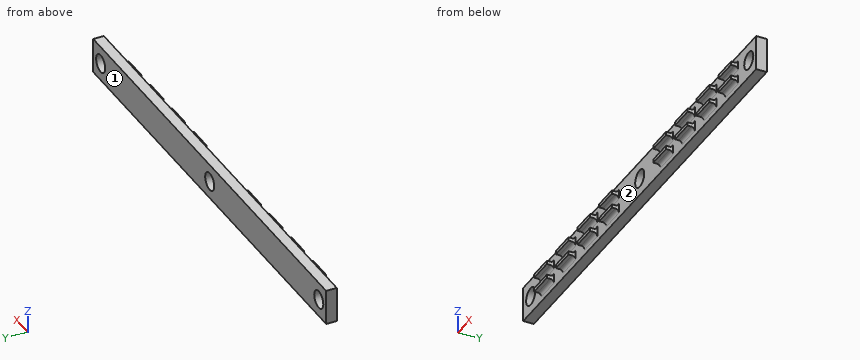
```python
from build123d import *

# Parameters (mm, degrees)
SKETCH1_W              = 129
SKETCH1_H              = 3
BOSS_EXTRUDE1_DEPTH    = 10
SKETCH2_R              = 2.5
CUT_EXTRUDE1_DEPTH     = 4
SKETCH3_W              = 7
SKETCH3_H              = 1
BOSS_EXTRUDE2_DEPTH    = 2
FILLET1_R              = 1
LPATTERN1_COUNT        = 4
LPATTERN1_PITCH        = 12
FILLET1_OF_LPATTERN1_R = 1


with BuildPart() as part:
    # Sketch1 → Boss-Extrude1 (new body)
    with BuildSketch(Plane.XY):
        with Locations((64.5, 1.5)):
            Rectangle(SKETCH1_W, SKETCH1_H)
    extrude(amount=BOSS_EXTRUDE1_DEPTH)

    # Sketch2 → Cut-Extrude1 (cut, through all)
    with BuildSketch(Plane.XZ):
        with Locations(Location((4.1, 5, 0), (0, 0, 270))):  # turned: the seam where the file's is
            Circle(SKETCH2_R)
        with Locations(Location((64.5, 5, 0), (0, 0, 270))):  # turned: the seam where the file's is
            Circle(SKETCH2_R)
        with Locations(Location((124.9, 5, 0), (0, 0, 270))):  # turned: the seam where the file's is
            Circle(SKETCH2_R)
    extrude(amount=-CUT_EXTRUDE1_DEPTH, mode=Mode.SUBTRACT)

    # Sketch3 → Boss-Extrude2 (add)
    with BuildSketch(Plane(origin=(0, 0, 0), x_dir=(1, 0, 0), z_dir=(0, 1, 0))):
        with Locations((13.5, -2.9)):
            Rectangle(SKETCH3_W, SKETCH3_H)
        with Locations((13.5, -7.1)):
            Rectangle(SKETCH3_W, SKETCH3_H)
        with Locations((79.5, -2.9)):
            Rectangle(SKETCH3_W, SKETCH3_H)
        with Locations((79.5, -7.1)):
            Rectangle(SKETCH3_W, SKETCH3_H)
    boss_extrude2 = extrude(amount=-BOSS_EXTRUDE2_DEPTH)

    # Fillet1
    fillet1_edges = [part.edges().sort_by_distance(p)[0] for p in [
        (13.5, 0, 3.4),
        (13.5, 0, 2.4),
        (13.5, 0, 7.6),
        (13.5, 0, 6.6),
        (79.5, 0, 3.4),
        (79.5, 0, 2.4),
        (79.5, 0, 7.6),
        (79.5, 0, 6.6),
    ]]
    fillet(fillet1_edges, radius=FILLET1_R)

    # LPattern1: Boss-Extrude2 ×4
    with Locations(*[(i * LPATTERN1_PITCH, 0, 0) for i in range(1, LPATTERN1_COUNT)]):
        add(boss_extrude2)

    # Fillet1 of LPattern1
    fillet1_of_lpattern1_edges = [part.edges().sort_by_distance(p)[0] for p in [
        (25.5, 0, 3.4),
        (25.5, 0, 2.4),
        (25.5, 0, 7.6),
        (25.5, 0, 6.6),
        (91.5, 0, 3.4),
        (91.5, 0, 2.4),
        (91.5, 0, 7.6),
        (91.5, 0, 6.6),
        (37.5, 0, 3.4),
        (37.5, 0, 2.4),
        (37.5, 0, 7.6),
        (37.5, 0, 6.6),
        (103.5, 0, 3.4),
        (103.5, 0, 2.4),
        (103.5, 0, 7.6),
        (103.5, 0, 6.6),
        (49.5, 0, 3.4),
        (49.5, 0, 2.4),
        (49.5, 0, 7.6),
        (49.5, 0, 6.6),
        (115.5, 0, 3.4),
        (115.5, 0, 2.4),
        (115.5, 0, 7.6),
        (115.5, 0, 6.6),
    ]]
    fillet(fillet1_of_lpattern1_edges, radius=FILLET1_OF_LPATTERN1_R)


solid = part.part
```
Could you check a few things on this model? Use its own coordinates, in mm. Face numbers are marked on the shaded views. Give positions to 0.01 mm unless a question says otherwise; leave off trailing zeros. Loops run counter-clockwise (first coordinate to the right, second up) from the corner with the lowest first, then second, coordinate; pieces in that order, holes last. Notation, with made-up numbers: (54.5, -27.75) - (82.5, -27.75) arc R10 ccw to (82.5, -20.75) - close; hole circle Ø1 at (23, 73.25). An arc over 180 degrees is marked (long way). Answer in a Markdown table with one row per item. Add a question column.
Q1. Please list where these lines run through material, in increasing order: L1, parallel to X at y = 2.45, z = 5; L2, parallel to X at y = 0.7, z = 7.25; L3, parallel to Y at x = 99, z = 5. Write a range as from..to.
Q2. If we section it at B-B (x = 93): List the corners of the cut face in (y, z) for me.
Q3. If we section it at A-A (x = 4.1): List the corners of the cut face in (y, z) for me, plus the area to 3 significant figures.
Q4. For pin 1 (0.5 mm diameter, centred on x = 25, y = -1.5, fed in from +Z); pin 2 (1.6 mm diameter, centred on y = -1.5, z = 7.5, fed in from +X); pin 3 (0.8 mm diameter, centred on x = 37, y = -1.5, fed in from -Z); pin 4 (4.5 mm diameter, centred on x = 124.9, z = 5, fed in from -Y), each with a flat end and sliding along its axis, tell me the tip position at first contact or that it passes through.
Q5. If we section it at C-C (x = 32): List the corners of the cut face in (y, z) for me.
Q6. We'd pull the mould along X, two halves only. Please class the marked faces 1 and 2: +X half, -X half, draft (parallel to the pull), parting line (faces both ways), or undercut.
The answers:
| question | item | result |
|---|---|---|
| 1 | L1 | x = 0..1.6, 6.6..62, 67..122.4, 127.4..129 |
| 1 | L2 | x = 0..3.01, 5.19..63.41, 65.59..123.81, 125.99..129 |
| 1 | L3 | y = 0..3 |
| 2 | outline | (-2, 2.4) - (-1, 2.4) arc R1 cw to (0, 1.4) - (0, 0) - (3, 0) - (3, 10) - (0, 10) - (0, 8.6) arc R1 cw to (-1, 7.6) - (-2, 7.6) - (-2, 6.6) - (-1, 6.6) arc R1 cw to (0, 5.6) - (0, 4.4) arc R1 cw to (-1, 3.4) - (-2, 3.4) - close |
| 3 | outline | (0, 0) - (3, 0) - (3, 2.5) - (0, 2.5) - close; (0, 7.5) - (3, 7.5) - (3, 10) - (0, 10) - close |
| 3 | area | 15.0 mm^2 |
| 4 | pin 1 | stops at z = 7.6 |
| 4 | pin 2 | stops at x = 119 |
| 4 | pin 3 | stops at z = 2.4 |
| 4 | pin 4 | passes through |
| 5 | outline | (0, 0) - (3, 0) - (3, 10) - (0, 10) - close |
| 6 | face 1 | draft |
| 6 | face 2 | undercut |
